```python
from build123d import *


with BuildPart() as part:
    # Sketch1 → Revolve1 (revolve)
    with BuildSketch(Plane.XY, mode=Mode.PRIVATE) as revolve1_sk:
        with BuildLine():
            Line((-1.4605, 0), (-1.4605, 12.065))
            Line((-1.4605, 12.065), (-2.2225, 12.065))
            ThreePointArc((-2.2225, 12.065), (-3.531586036, 11.903844145), (-4.7625, 11.43))
            Line((-4.7625, 11.43), (-4.7625, 10.795))
            ThreePointArc((-4.7625, 10.795), (-4.688105122, 10.615394878), (-4.5085, 10.541))
            Line((-4.5085, 10.541), (-2.39395, 10.541))
            Line((-2.39395, 10.541), (-2.39395, 0))
            Line((-2.39395, 0), (-1.4605, 0))
        make_face()
    revolve(revolve1_sk.sketch.rotate(Axis((0, 0, 0), (0, 1, 0)), 270), axis=Axis((0, 0, 0), (0, 1, 0)))


solid = part.part
```
Input: part model. Units: mm. Frame: model coordinates. A direction names the side the tool comes from. Give positions to 0.01 mm unless a question says otherwise; leave off trailing zeros. Loops run counter-clockwise (first coordinate to the right, second up) from the corner with the lowest first, then second, coordinate; pieces in that order, holes last. Notation, with made-up numbers: M 56,16 L 85,16 A21 cw 85,48 Z; hole C 38.5,48.5 d3. An arc over 180 degrees is marked long. Answer as CSV lines item,"result". Start each with the question number.
1. Pin query (flat end, axial travel): P1, Ø4, axis at y = 9, z = 0, coming from the -X side; P2, Ø1.5, axis at x = 0.5, y = 8, coming from the -Z side; P3, Ø2.5, axis at x = 0, z = 0, coming from the -Y side; P4, Ø1.5, axis at x = 3, z = -2, coming from the -Y side. Return the tip coordinate at first contact, or that it passes through.
2. Reachability of faces 4 (the face through (2, 10.541, -2)), 5 (the face through (-2, 12.065, 0)) from +Z, -Z, +X, -X, +Y, -Y: full face, straight path, thin tool, end or side. Return the list, or none.
3. Section A-A on y = 3. Return loops of the section in (x, z).
4. Pull-direction query (Z, two-part tool) for faces 1 (the face through (0.89, 6.12, 1.16)), 2 (the face through (2, 0, 0)), 3 (the face through (-0.719, 5.197, -2.283)); classes: released by +Z, released by -Z, zero draft, split by the parting line, or undercut.
5. Line query: L1, parallel to X at y = 3.75, z = 0; L2, parallel to X at y = 2.5, z = -0.5; L3, parallel to Z at x = -0.75, y = 8. Output: solid intervals per line, ascending.
Computed values:
1,P1,"stops at x = -4.76"
1,P2,"stops at z = -2.39"
1,P3,"passes through"
1,P4,"stops at y = 10.54"
2,face 4,"-Y"
2,face 5,"+Z, -Z, +X, -X, +Y"
3,outline,"C 0,0 d4.79; hole C 0,0 d2.92"
4,face 1,"undercut"
4,face 2,"zero draft"
4,face 3,"split by the parting line"
5,L1,"x = -2.39 to -1.46, 1.46 to 2.39"
5,L2,"x = -2.34 to -1.37, 1.37 to 2.34"
5,L3,"z = -2.27 to -1.25, 1.25 to 2.27"
